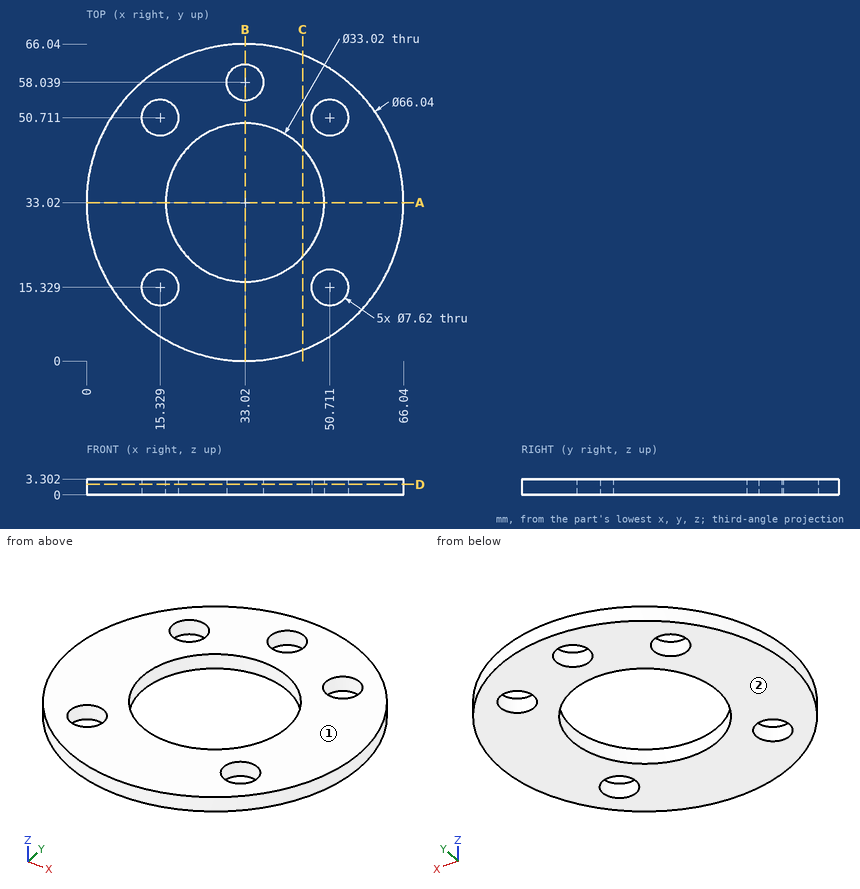
Here's the drawing with two shaded views (mm, measured from the low corner). I have some questions. Round coordinates to 2 decimals unless told otherwise and drop trailing zeros. Order: outer loops, then holes, each group sorted by start corner. A loop starts at its lowest first (then second) coordinate and runs counter-clockwise, first axis right, second up. Notation, with made-up numbers: (60, 49) -> (65, 49) arc R12 cw to (65, 59) -> close; hole circle Ø1 at (73.25, 74). An arc over 180 degrees is marked (long way). Use a Markdown table: item, result. Add a question column.
(1) Suppose I cut it at C-C, the plane x = 45. Please give me the cut outline in (y, z).
(2) Suppose I cut it at A-A, the plane y = 33.02. Please give me the cut outline in (x, z), and give its area (3 significant figures).
(3) If we mould it in two halves opening along Z, with no side actions, what happens to the marked faces 1 and 2? For each: released by +Z, released by -Z, zero draft, split by the parting line, or undercut.
(4) Suppose I cut it at B-B, the plane x = 33.02. Please give me the cut outline in (y, z), and give its area (3 significant figures).
(5) I need wall thicknesses on line 1 along Y through (x, z) = (33.02, 0.9); line 2 along X through (y, z) = (33, 1.9); line 3 along Y through (x, z) = (51.5, 2.2). Which ranges of each line are inside material? Lowest first, please.
(6) Suppose I cut it at D-D, the plane z = 2.2. Please give me the cut outline in (x, y).
Verdict:
| question | item | result |
|---|---|---|
| 1 | outline | (2.25, 0) -> (21.66, 0) -> (21.66, 3.3) -> (2.25, 3.3) -> close; (44.38, 0) -> (63.79, 0) -> (63.79, 3.3) -> (44.38, 3.3) -> close |
| 2 | outline | (0, 0) -> (16.51, 0) -> (16.51, 3.3) -> (0, 3.3) -> close; (49.53, 0) -> (66.04, 0) -> (66.04, 3.3) -> (49.53, 3.3) -> close |
| 2 | area | 109 mm2 |
| 3 | face 1 | released by +Z |
| 3 | face 2 | released by -Z |
| 4 | outline | (0, 0) -> (16.51, 0) -> (16.51, 3.3) -> (0, 3.3) -> close; (49.53, 0) -> (54.23, 0) -> (54.23, 3.3) -> (49.53, 3.3) -> close; (61.85, 0) -> (66.04, 0) -> (66.04, 3.3) -> (61.85, 3.3) -> close |
| 4 | area | 83.9 mm2 |
| 5 | line 1 | 0 to 16.51, 49.53 to 54.23, 61.85 to 66.04 |
| 5 | line 2 | 0 to 16.51, 49.53 to 66.04 |
| 5 | line 3 | 5.66 to 11.6, 19.06 to 46.98, 54.44 to 60.38 |
| 6 | outline | circle Ø66.04 at (33.02, 33.02); hole circle Ø7.62 at (15.33, 15.33); hole circle Ø7.62 at (15.33, 50.71); hole circle Ø33.02 at (33.02, 33.02); hole circle Ø7.62 at (33.02, 58.04); hole circle Ø7.62 at (50.71, 15.33); hole circle Ø7.62 at (50.71, 50.71) |
